Source: three-view drawing plus pictorial views. Frame: mm from the lowest corner of the part. Give positions to 0.01 mm unless a question says otherwise; leave off trailing zeros. Write each loop counter-clockwise with the first axis right and the second up, starting at its lowest first coordinate (ties: lowest second). Pieces come first, ordered by that corner, then holes.
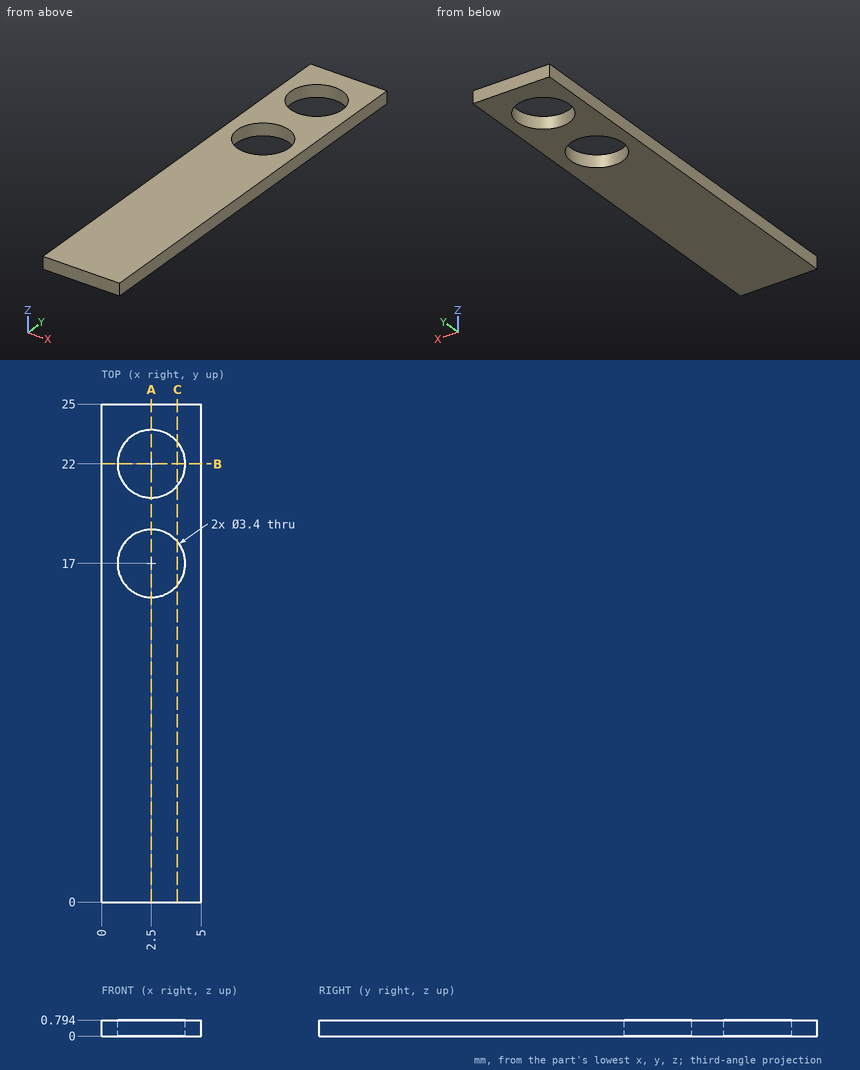
Q1. Ray query, line 1 along Y through (x, z) = (2.5, 0.1); line 2 along Y through (x, z) = (3.75, 0.75); line 3 along X through (y, z) = (17.5, 0.1) (1 decimal). Return the intervals inside material, ascending.
Filled sheet:
line 1: y = 0 to 15.3, 18.7 to 20.3, 23.7 to 25
line 2: y = 0 to 15.85, 18.15 to 20.85, 23.15 to 25
line 3: x = 0 to 0.9, 4.1 to 5
Q2. Section A-A on x = 2.5. Output: boundary loops of the cut face in (y, z).
Filled sheet:
outline: (0, 0) - (15.3, 0) - (15.3, 0.79) - (0, 0.79) - close; (18.7, 0) - (20.3, 0) - (20.3, 0.79) - (18.7, 0.79) - close; (23.7, 0) - (25, 0) - (25, 0.79) - (23.7, 0.79) - close
Q3. Section B-B on y = 22. Output: boundary loops of the cut face in (x, z).
Filled sheet:
outline: (0, 0) - (0.8, 0) - (0.8, 0.79) - (0, 0.79) - close; (4.2, 0) - (5, 0) - (5, 0.79) - (4.2, 0.79) - close
Q4. Section C-C on x = 3.8. Output: boundary loops of the cut face in (y, z) (1 decimal).
Filled sheet:
outline: (0, 0) - (15.9, 0) - (15.9, 0.8) - (0, 0.8) - close; (18.1, 0) - (20.9, 0) - (20.9, 0.8) - (18.1, 0.8) - close; (23.1, 0) - (25, 0) - (25, 0.8) - (23.1, 0.8) - close
Q5. Pin query (flat end, axial travel): P1, Ø3, axis at x = 1, y = 22, coming from the -Z side; P2, Ø3, axis at x = 2.5, y = 17, coming from the +Z side. Return the tip coordinate at first contact, or that it passes through.
Filled sheet:
P1: stops at z = 0
P2: passes through
